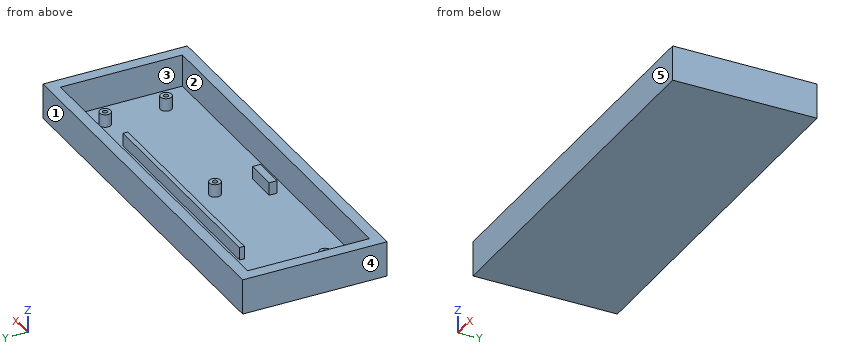
```python
from build123d import *

# Parameters (mm, degrees)
SKETCH_W         = 240
SKETCH_H         = 90
PAD_DEPTH        = 10
SKETCH001_W      = 225
SKETCH001_H      = 76
SKETCH001_R      = 3.5
SKETCH001_W_2    = 140
SKETCH001_H_2    = 3
SKETCH001_W_3    = 20
SKETCH001_H_3    = 5
SKETCH001_R_2    = 1.5
POCKET_DEPTH     = 8
POCKET_FACE5_W   = 90
POCKET_FACE5_H   = 240
POCKET_FACE5_W_2 = 76
POCKET_FACE5_H_2 = 225
PAD001_DEPTH     = 12


with BuildPart() as part:
    # Sketch → Pad (new body)
    with BuildSketch(Plane.XY):
        Rectangle(SKETCH_W, SKETCH_H)
    extrude(amount=PAD_DEPTH)

    # Sketch001 (on Face6 of Pad) → Pocket (cut)
    with BuildSketch(Plane.XY.offset(10)):
        Rectangle(SKETCH001_W, SKETCH001_H)
        Circle(SKETCH001_R, mode=Mode.SUBTRACT)
        with Locations((-95.5, -19)):
            Circle(SKETCH001_R, mode=Mode.SUBTRACT)
        with Locations((95.5, 19)):
            Circle(SKETCH001_R, mode=Mode.SUBTRACT)
        with Locations((95.5, -19)):
            Circle(SKETCH001_R, mode=Mode.SUBTRACT)
        with Locations((0, 19.5)):
            Rectangle(SKETCH001_W_2, SKETCH001_H_2, mode=Mode.SUBTRACT)
        with Locations((-5, -28.5)):
            Rectangle(SKETCH001_W_3, SKETCH001_H_3, mode=Mode.SUBTRACT)
        with Locations((-95.5, -19)):
            Circle(SKETCH001_R_2)
        with Locations((95.5, 19)):
            Circle(SKETCH001_R_2)
        with Locations((95.5, -19)):
            Circle(SKETCH001_R_2)
        Circle(SKETCH001_R_2)
    extrude(amount=-POCKET_DEPTH, mode=Mode.SUBTRACT)

    # Pocket Face5 → Pad001 (add)
    with BuildSketch(Plane(origin=(0, 0, 10), x_dir=(0, 1, 0), z_dir=(0, 0, 1))):
        Rectangle(POCKET_FACE5_W, POCKET_FACE5_H)
        Rectangle(POCKET_FACE5_W_2, POCKET_FACE5_H_2, mode=Mode.SUBTRACT)
    extrude(amount=PAD001_DEPTH)


solid = part.part
```
Model file for the job. Use its own axes, mm. Face numbers are marked on the shaded views. A direction names the side the tool comes from. Round coordinates to 2 decimals unless told otherwise and drop trailing zeros. Write each loop counter-clockwise with the first axis right and the second up, starting at its lowest first coordinate (ties: lowest second). Pieces come first, ordered by that corner, then holes. Notation, with made-up numbers: (58, -8.5) - (75, -8.5) arc R35 ccw to (75, 29.5) - close; hole circle Ø6 at (0.5, 7). An arc over 180 degrees is marked (long way). Use CSV: the item, a comma, the result in double quotes. Start each with the question number.
Item 1: Drill centre lines: L1, parallel to Y at x = -95.5, z = 6.5; L2, parallel to Y at x = 77.5, z = 2.75; L3, parallel to X at y = -2, z = 14.5. Where is each one in solid material? Low to high. Write a range as [from, to].
Item 2: Pin check, flat tips, straight feed: P1, Ø5.5, axis at x = -95, y = -20.5, coming from the +Z side; P2, Ø1.5, axis at x = -0.5, y = 0.5, coming from the +Z side. Stop position of each tip, or through.
Item 3: Band-saw the part on A-A (z = 7.75). State how many separate pieces and enclosed holes the cut face has, and give its area (3 significant figures).
Item 4: Band-saw the part on D-D (x = 104). Write the cut outline in (y, z).
Item 5: Band-saw the part on B-B (x = 35.5). Write the cut outline in (y, z).
Item 6: Two-plate mould, pull along Y, no slides. Class the marked faces 3, 4 and 5: released by +Y, released by -Y, zero draft, split by the parting line, or undercut.
Item 7: Tool access for the marked faces 1 and 2: list every direction of +Z, -Z, +X, -X, +Y, -Y with a clear straight run to the whole face (end or side of a thin tool).
Item 8: Band-saw the part on C-C (y = 28). Write the cut outline in (x, z), and give its area (3 significant figures).
Checked values:
1,L1,"y = [-45, -38], [-22.5, -20.5], [-17.5, -15.5], [38, 45]"
1,L2,"y = [-45, -38], [38, 45]"
1,L3,"x = [-120, -112.5], [112.5, 120]"
2,P1,"stops at z = 10"
2,P2,"stops at z = 2"
3,separate pieces,"7"
3,enclosed holes,"5"
3,area,"5,150 mm²"
4,outline,"(-45, 0) - (45, 0) - (45, 22) - (38, 22) - (38, 2) - (-38, 2) - (-38, 22) - (-45, 22) - close"
5,outline,"(-45, 0) - (45, 0) - (45, 22) - (38, 22) - (38, 2) - (21, 2) - (21, 10) - (18, 10) - (18, 2) - (-38, 2) - (-38, 22) - (-45, 22) - close"
6,face 3,"undercut"
6,face 4,"zero draft"
6,face 5,"released by -Y"
7,face 1,"+Z, -Z, +X, -X, +Y"
7,face 2,"+Z"
8,outline,"(-120, 0) - (120, 0) - (120, 22) - (112.5, 22) - (112.5, 2) - (-112.5, 2) - (-112.5, 22) - (-120, 22) - close"
8,area,"780 mm²"
